Here's how the part is built. I have some questions about the finished solid (model axes, mm). A direction names the side the tool comes from. Coordinates: 2 decimals unless noted, no trailing zeros. Order: outer loops, then holes, each group sorted by start corner. A loop starts at its lowest first (then second) coordinate and runs counter-clockwise, first axis right, second up. Notation, with made-up numbers: M -29.75,47.25 L 17.25,47.25 A11 ccw 17.25,67.25 Z; hole C 85.5,28 d3. An arc over 180 degrees is marked long. One line per question, with ' | ' between items. Start each with the question number.
```python
from build123d import *

# Parameters (mm, degrees)
EXTRUDE_1_DEPTH      = 3
SKETCH_2_R           = 1.75
CUT_EXTRUDE_1_DEPTH  = 10
CUT_EXTRUDE_2_DEPTH  = 10
CUT_EXTRUDE_3_DEPTH  = 10
SKETCH_5_R           = 1.75
CUT_EXTRUDE_4_DEPTH  = 10
SKETCH_6_R           = 1.65
CUT_EXTRUDE_5_DEPTH  = 10
CUT_EXTRUDE_8_DEPTH  = 10
CUT_EXTRUDE_9_DEPTH  = 10
CUT_EXTRUDE_10_DEPTH = 10


with BuildPart() as part:
    # 草图1 → 凸台-拉伸1 (new body)
    with BuildSketch(Plane(origin=(0, 0, 0), x_dir=(1, 0, 0), z_dir=(0, 1, 0))):
        with BuildLine():
            Line((-66.78059141, 154.593992167), (66.78059141, 154.593992167))
            ThreePointArc((66.78059141, 154.593992167), (85.265515034, 148.222525736), (95.898700635, 131.814498742))
            Line((95.898700635, 131.814498742), (111.265547961, 69.844672358))
            ThreePointArc((111.265547961, 69.844672358), (112.147438737, 62.624165782), (111.265547961, 55.403659207))
            Line((111.265547961, 55.403659207), (95.898700635, -6.566167178))
            ThreePointArc((95.898700635, -6.566167178), (85.265515034, -22.974194171), (66.78059141, -29.345660602))
            Line((66.78059141, -29.345660602), (-66.78059141, -29.345660602))
            ThreePointArc((-66.78059141, -29.345660602), (-85.265515034, -22.974194171), (-95.898700635, -6.566167178))
            Line((-95.898700635, -6.566167178), (-111.265547961, 55.403659207))
            ThreePointArc((-111.265547961, 55.403659207), (-112.147438737, 62.624165782), (-111.265547961, 69.844672358))
            Line((-111.265547961, 69.844672358), (-95.898700635, 131.814498742))
            ThreePointArc((-95.898700635, 131.814498742), (-85.265515034, 148.222525736), (-66.78059141, 154.593992167))
        make_face()
    extrude(amount=EXTRUDE_1_DEPTH)

    # 草图2 → 切除-拉伸1 (cut)
    with BuildSketch(Plane(origin=(0, 3, 0), x_dir=(1, 0, 0), z_dir=(0, 1, 0))):
        with Locations(Location((104.507530951, 62.624165782, 0), (0, 0, 270))):
            Circle(SKETCH_2_R)
        with Locations(Location((80.450184708, -16.818951307, 0), (0, 0, 270))):
            Circle(SKETCH_2_R)
        with Locations(Location((-80.450184708, -16.818951307, 0), (0, 0, 270))):
            Circle(SKETCH_2_R)
        with Locations(Location((-104.507530951, 62.624165782, 0), (0, 0, 270))):
            Circle(SKETCH_2_R)
        with Locations(Location((0, 144.079729864, 0), (0, 0, 270))):
            Circle(SKETCH_2_R)
        with Locations(Location((0, 131.568155221, 0), (0, 0, 270))):
            Circle(SKETCH_2_R)
    extrude(amount=-CUT_EXTRUDE_1_DEPTH, mode=Mode.SUBTRACT)

    # 草图3 → 切除-拉伸2 (cut)
    with BuildSketch(Plane(origin=(0, 3, 0), x_dir=(1, 0, 0), z_dir=(0, 1, 0))):
        with BuildLine():
            Line((14.696938457, 59.265841846), (44.774939174, 29.187841128))
            ThreePointArc((44.774939174, 29.187841128), (45.652778395, 26.995514412), (44.672172354, 24.847187174))
            ThreePointArc((44.672172354, 24.847187174), (0, 7.570427798), (-44.672172354, 24.847187174))
            ThreePointArc((-44.672172354, 24.847187174), (-45.652778395, 26.995514412), (-44.774939174, 29.187841128))
            Line((-44.774939174, 29.187841128), (-14.696938457, 59.265841846))
            ThreePointArc((-14.696938457, 59.265841846), (-12.790455415, 60.136819103), (-10.77910124, 59.547129902))
            ThreePointArc((-10.77910124, 59.547129902), (0, 55.962780302), (10.77910124, 59.547129902))
            ThreePointArc((10.77910124, 59.547129902), (12.790455415, 60.136819103), (14.696938457, 59.265841846))
        make_face()
    extrude(amount=-CUT_EXTRUDE_2_DEPTH, mode=Mode.SUBTRACT)

    # 草图4 → 切除-拉伸3 (cut)
    with BuildSketch(Plane(origin=(0, 3, 0), x_dir=(1, 0, 0), z_dir=(0, 1, 0))):
        with BuildLine():
            Line((-36.857879598, 37.104900704), (-60.429301447, 13.533478855))
            ThreePointArc((-60.429301447, 13.533478855), (-61.599780589, 10.611517412), (-60.293966994, 7.747476395))
            ThreePointArc((-60.293966994, 7.747476395), (0, -15.59071727), (60.293966994, 7.747476395))
            ThreePointArc((60.293966994, 7.747476395), (61.599780589, 10.611517412), (60.429301447, 13.533478855))
            Line((60.429301447, 13.533478855), (36.857879598, 37.104900704))
            Line((36.857879598, 37.104900704), (-36.857879598, 37.104900704))
        make_face()
    extrude(amount=-CUT_EXTRUDE_3_DEPTH, mode=Mode.SUBTRACT)

    # 草图5 → 切除-拉伸4 (cut)
    with BuildSketch(Plane(origin=(0, 3, 0), x_dir=(1, 0, 0), z_dir=(0, 1, 0))):
        with Locations(Location((47.527679448, 141.148627896, 0), (0, 0, 270))):
            Circle(SKETCH_5_R)
        with Locations(Location((-46.069524323, 84.050974576, 0), (0, 0, 270))):
            Circle(SKETCH_5_R)
        with Locations(Location((-46.069524323, 141.148627896, 0), (0, 0, 270))):
            Circle(SKETCH_5_R)
    extrude(amount=-CUT_EXTRUDE_4_DEPTH, mode=Mode.SUBTRACT)

    # 草图6 → 切除-拉伸5 (cut)
    with BuildSketch(Plane(origin=(0, 3, 0), x_dir=(1, 0, 0), z_dir=(0, 1, 0))):
        with Locations(Location((65.550657258, 102.864758009, 0), (0, 0, 270))):
            Circle(SKETCH_6_R)
        with Locations(Location((91.050657258, 102.864758009, 0), (0, 0, 270))):
            Circle(SKETCH_6_R)
        with Locations(Location((91.050657258, 85.864758009, 0), (0, 0, 270))):
            Circle(SKETCH_6_R)
        with Locations(Location((65.550657258, 85.864758009, 0), (0, 0, 270))):
            Circle(SKETCH_6_R)
    extrude(amount=-CUT_EXTRUDE_5_DEPTH, mode=Mode.SUBTRACT)

    # 草图7 → 切除-拉伸8 (cut)
    with BuildSketch(Plane(origin=(0, 3, 0), x_dir=(1, 0, 0), z_dir=(0, 1, 0))):
        with BuildLine():
            Line((-11.016648097, -20.513898252), (11.016648097, -20.513898252))
            ThreePointArc((11.016648097, -20.513898252), (13.814702514, -21.911306641), (14.378457093, -24.987674549))
            add(Edge.make_bspline(
                [(14.378457093, -24.987674549), (14.050661547, -26.11933694), (10.489346867, -26.76009099), (7.724749574, -26.493757466), (5.904508816, -27.417302496), (5.804576355, -27.473305111)],
                knots=[0, 0, 0, 0, 0.274123853, 0.745489655, 0.777393608, 0.777393608, 0.777393608, 0.777393608], degree=3))
            ThreePointArc((5.804576355, -27.473305111), (5.325885634, -28.59829127), (6.293448421, -29.345660602))
            Line((6.293448421, -29.345660602), (8.755585002, -29.345660602))
            Line((8.755585002, -29.345660602), (8.755585002, -31.412448424))
            Line((8.755585002, -31.412448424), (-8.755585002, -31.412448424))
            Line((-8.755585002, -31.412448424), (-8.755585002, -29.804465611))
            Line((-8.755585002, -29.804465611), (-8.755585002, -29.345660602))
            Line((-8.755585002, -29.345660602), (-6.293448421, -29.345660602))
            ThreePointArc((-6.293448421, -29.345660602), (-5.325885634, -28.59829127), (-5.804576355, -27.473305111))
            add(Edge.make_bspline(
                [(-14.378457093, -24.987674549), (-14.050661547, -26.11933694), (-10.489346867, -26.76009099), (-7.724749574, -26.493757466), (-5.904508816, -27.417302496), (-5.804576355, -27.473305111)],
                knots=[0, 0, 0, 0, 0.274123853, 0.745489655, 0.777393608, 0.777393608, 0.777393608, 0.777393608], degree=3))
            ThreePointArc((-14.378457093, -24.987674549), (-13.814702514, -21.911306641), (-11.016648097, -20.513898252))
        make_face()
    extrude(amount=-CUT_EXTRUDE_8_DEPTH, mode=Mode.SUBTRACT)

    # 草图8 → 切除-拉伸9 (cut)
    with BuildSketch(Plane(origin=(0, 3, 0), x_dir=(1, 0, 0), z_dir=(0, 1, 0))):
        with BuildLine():
            Line((-31.230806012, 58.302254227), (-63.873737866, 25.659322373))
            ThreePointArc((-63.873737866, 25.659322373), (-66.3486116, 25.659322373), (-66.3486116, 28.134196107))
            Line((-66.3486116, 28.134196107), (-33.705679746, 60.777127961))
            ThreePointArc((-33.705679746, 60.777127961), (-31.230806012, 60.777127961), (-31.230806012, 58.302254227))
        make_face()
        with BuildLine():
            Line((-37.026832233, 64.098280448), (-69.669764087, 31.455348594))
            ThreePointArc((-69.669764087, 31.455348594), (-72.144637821, 31.455348594), (-72.144637821, 33.930222328))
            Line((-72.144637821, 33.930222328), (-39.501705967, 66.573154182))
            ThreePointArc((-39.501705967, 66.573154182), (-37.026832233, 66.573154182), (-37.026832233, 64.098280448))
        make_face()
        with BuildLine():
            Line((37.026832233, 64.098280448), (69.669764087, 31.455348594))
            ThreePointArc((69.669764087, 31.455348594), (72.144637821, 31.455348594), (72.144637821, 33.930222328))
            Line((72.144637821, 33.930222328), (39.501705967, 66.573154182))
            ThreePointArc((39.501705967, 66.573154182), (37.026832233, 66.573154182), (37.026832233, 64.098280448))
        make_face()
        with BuildLine():
            Line((31.230806012, 58.302254227), (63.873737866, 25.659322373))
            ThreePointArc((63.873737866, 25.659322373), (66.3486116, 25.659322373), (66.3486116, 28.134196107))
            Line((66.3486116, 28.134196107), (33.705679746, 60.777127961))
            ThreePointArc((33.705679746, 60.777127961), (31.230806012, 60.777127961), (31.230806012, 58.302254227))
        make_face()
    extrude(amount=-CUT_EXTRUDE_9_DEPTH, mode=Mode.SUBTRACT)

    # 草图9 → 切除-拉伸10 (cut)
    with BuildSketch(Plane(origin=(0, 3, 0), x_dir=(1, 0, 0), z_dir=(0, 1, 0))):
        with BuildLine():
            Line((-3.845016723, 66.126250856), (3.845016723, 66.126250856))
            ThreePointArc((3.845016723, 66.126250856), (5.919206434, 59.807077742), (7.993396144, 66.126250856))
            Line((7.993396144, 66.126250856), (11.658238607, 66.126250856))
            Line((11.658238607, 66.126250856), (11.658238607, 110.119100398))
            Line((11.658238607, 110.119100398), (7.806916331, 110.119100398))
            ThreePointArc((7.806916331, 110.119100398), (5.919206434, 116.566395996), (4.031496536, 110.119100398))
            Line((4.031496536, 110.119100398), (-4.031496536, 110.119100398))
            ThreePointArc((-4.031496536, 110.119100398), (-5.919206434, 116.566395996), (-7.806916331, 110.119100398))
            Line((-7.806916331, 110.119100398), (-11.930882282, 110.119100398))
            Line((-11.930882282, 110.119100398), (-11.930882282, 66.126250856))
            Line((-11.930882282, 66.126250856), (-7.993396144, 66.126250856))
            ThreePointArc((-7.993396144, 66.126250856), (-5.919206434, 59.807077742), (-3.845016723, 66.126250856))
        make_face()
    extrude(amount=-CUT_EXTRUDE_10_DEPTH, mode=Mode.SUBTRACT)


solid = part.part
```
1. Imagine slicing it at A-A (z = -16.5). List the corners of the cut face in (x, y) for me, then the cut area to 3 significant figures.
2. Imagine slicing it at D-D (z = -93). List the corners of the cut face in (x, y) for me, then the cut area to 3 significant figures.
3. Will these pins go through, and if not, where does the flat tip stop? pin 1 (1.5 mm diameter, centred on y = 0.5, z = -53, fed in from +X); pin 2 (1 mm diameter, centred on y = 1, z = -57, fed in from -X).
4. Which directions (+Z, -Z, +X, -X, +Y, -Y) give clear straight access to the entire face, cutting with the end or side of a thin tool? Please do faces 1 (the face through (-0.926, 1.521, 15.586)), 2 (the face through (85.484, 1.479, 22.801)).
5. Imagine slicing it at B-B (x = -53). List the corners of the cut face in (y, z) for me.
6. We'd pull the mould along Z, two halves only. Please class faces 3 (the face through (2, 3, -64)), 4 (the face through (103.7, 1.5, -24.9)), 5 (the face through (-53.12, 1.521, -48.005)), 6 (the face through (-85.484, 1.479, -148.05)): released by +Z, released by -Z, zero draft, split by the parting line, or undercut.
7. Imagine slicing it at C-C (y = 1.3). Count the separate pieces of the cut face and the enclosed holes in it, then the cut area to 3 significant figures.
8. I need wall thicknesses on line 1 (Z direction, x = 60, y = 0.6); line 2 (Z direction, x = -59.5, y = 1.15); line 3 (X direction, y = 1.15, z = -34.5). Which ranges of each line are inside material? Lowest first, please.
Entries:
1) outline: M -101.62,0 L -57.46,0 L -57.46,3 L -101.62,3 Z; M 57.46,0 L 101.62,0 L 101.62,3 L 57.46,3 Z | area: 265 mm²
2) outline: M -105.52,0 L -11.93,0 L -11.93,3 L -105.52,3 Z; M 11.66,0 L 105.52,0 L 105.52,3 L 11.66,3 Z | area: 562 mm²
3) pin 1: x = 110.86 | pin 2: x = -111.71
4) face 1: +Y, -Y | face 2: +Z, +X, +Y, -Y
5) outline: M 0,-154.59 L 3,-154.59 L 3,-53.07 L 0,-53.07 Z; M 0,-48.13 L 3,-48.13 L 3,-41.48 L 0,-41.48 Z; M 0,-36.53 L 3,-36.53 L 3,-20.96 L 0,-20.96 Z; M 0,-1.78 L 3,-1.78 L 3,29.35 L 0,29.35 Z
6) face 3: zero draft | face 4: released by +Z | face 5: undercut | face 6: released by -Z
7) separate pieces: 1 | enclosed holes: 19 | area: 28,700 mm²
8) line 1: -154.59 to -46.07, -41.13 to -34.48, -29.53 to -13.96, -7.48 to 29.35 | line 2: -154.59 to -46.57, -41.63 to -34.98, -30.03 to -14.46, -7.03 to 29.35 | line 3: -106.08 to -71.57, -66.63 to -59.98, -55.03 to -39.46, 39.46 to 55.03, 59.98 to 66.63, 71.57 to 106.08
